Here's the drawing with two shaded views (mm, measured from the low corner). I have some questions. Give positions to 0.01 mm unless a question says otherwise; leave off trailing zeros. Loops run counter-clockwise (first coordinate to the right, second up) from the corner with the lowest first, then second, coordinate; pieces in that order, holes last. Notation, with made-up numbers: (68, 14) -> (119, 14) arc R14 cw to (119, 35) -> close; hole circle Ø4 at (33.25, 42.5). An arc over 180 degrees is marked (long way). Write each question's results on one line, items separated by ' | '. Start each with the question number.
Q1. If I drill on line 1 along X through (y, z) = (4.75, 1.75); line 2 along X through (y, z) = (2.5, 4.75); line 3 along X through (y, z) = (3, 2.25), over which ranges is the centre line in solid material (lowest first)?
Q2. We'd pull the mould along Y, two halves only. Please class the marked faces 1, 2, 3 and 4: released by +Y, released by -Y, zero draft, split by the parting line, or undercut.
Q3. If we section it at A-A, the plane x = 7: List the corners of the cut face in (y, z) for me (3 decimals), plus the area to 4 significant figures.
Q4. If we section it at D-D, the plane z = 9.25: List the corners of the cut face in (x, y) for me (3 decimals), plus the area to 3 significant figures.
Q5. If we section it at B-B, the plane z = 5.1: List the corners of the cut face in (x, y) for me (3 decimals).
Q6. If we section it at C-C, the plane y = 2: List the corners of the cut face in (x, z) for me.
Q7. Will this pin go through, and if not, where does the flat tip stop? P1, Ø0.6, axis at x = 22.5, z = 1, coming from the -Y side.
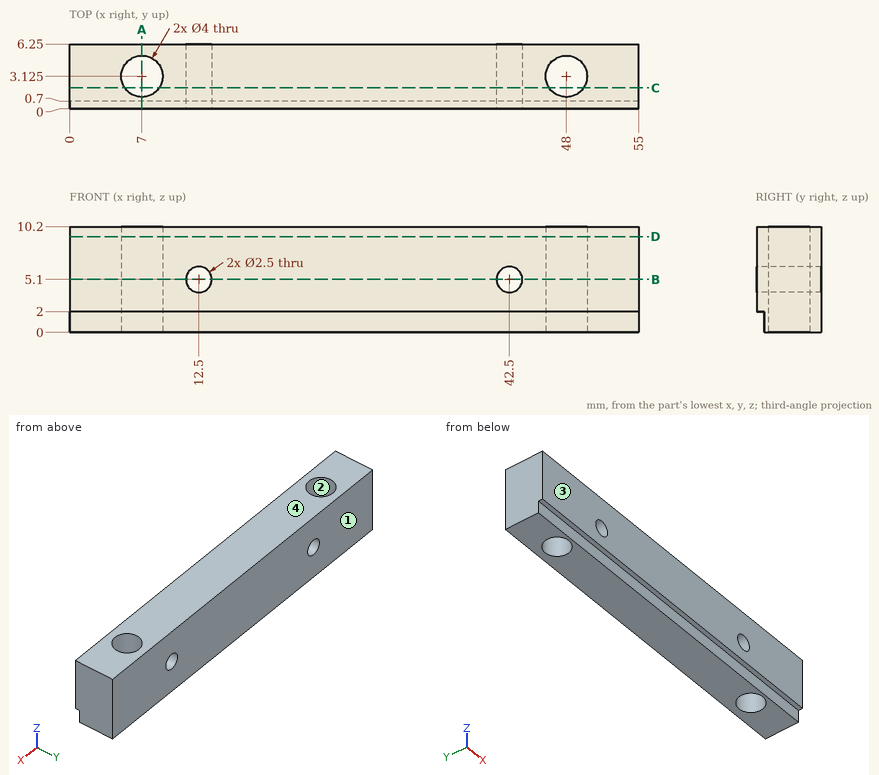
Final values:
1) line 1: x = 0 to 5.83, 8.17 to 46.83, 49.17 to 55 | line 2: x = 0 to 5.1, 8.9 to 11.3, 13.7 to 41.3, 43.7 to 46.1, 49.9 to 55 | line 3: x = 0 to 5, 9 to 46, 50 to 55
2) face 1: released by +Y | face 2: undercut | face 3: released by -Y | face 4: zero draft
3) outline: (0, 2) -> (0.7, 2) -> (0.7, 0) -> (1.125, 0) -> (1.125, 10.2) -> (0, 10.2) -> close; (5.125, 0) -> (6.25, 0) -> (6.25, 10.2) -> (5.125, 10.2) -> close | area: 21.55 mm²
4) outline: (0, 0) -> (55, 0) -> (55, 6.25) -> (0, 6.25) -> close; hole circle Ø4 at (7, 3.125); hole circle Ø4 at (48, 3.125) | area: 319 mm²
5) outline: (0, 0) -> (11.25, 0) -> (11.25, 6.25) -> (0, 6.25) -> close; (13.75, 0) -> (41.25, 0) -> (41.25, 6.25) -> (13.75, 6.25) -> close; (43.75, 0) -> (55, 0) -> (55, 6.25) -> (43.75, 6.25) -> close; hole circle Ø4 at (7, 3.125); hole circle Ø4 at (48, 3.125)
6) outline: (0, 0) -> (5.35, 0) -> (5.35, 10.2) -> (0, 10.2) -> close; (8.65, 0) -> (46.35, 0) -> (46.35, 10.2) -> (8.65, 10.2) -> close; (49.65, 0) -> (55, 0) -> (55, 10.2) -> (49.65, 10.2) -> close; hole circle Ø2.5 at (12.5, 5.1); hole circle Ø2.5 at (42.5, 5.1)
7) P1: stops at y = 0.7
